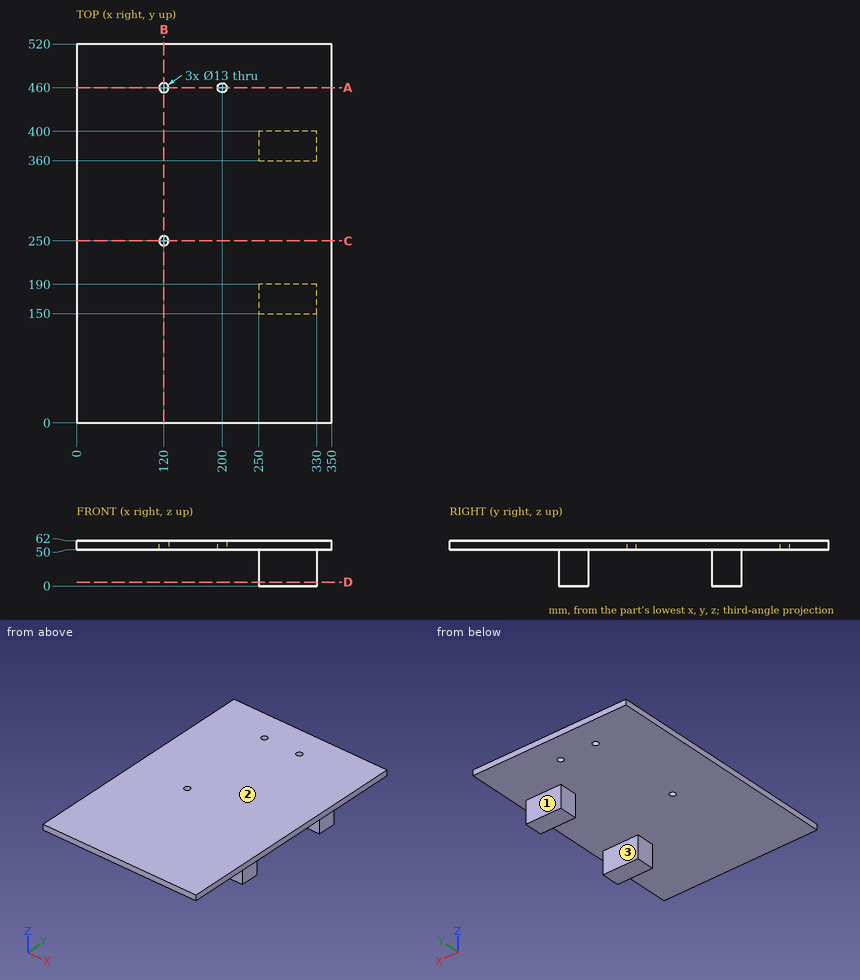
Input: dimensioned drawing with shaded views. Units: mm. Origin: part minimum x, y, z. Round coordinates to 2 decimals unless told otherwise and drop trailing zeros. Loops run counter-clockwise (first coordinate to the right, second up) from the corner with the lowest first, then second, coordinate; pieces in that order, holes last. Notation, with made-up numbers: M -2.75,3 L 50.25,3 A23 ccw 50.25,15 Z; hole C 20.5,-8 d10. An arc over 180 degrees is marked long. Return JSON: item names as keys, results as strings. Group by question number.
1. Section query A-A on y = 460. Output: boundary loops of the cut face in (x, z), and give its area (3 significant figures).
2. Section query B-B on x = 120. Output: boundary loops of the cut face in (y, z), and give its area (3 significant figures).
3. Section query D-D on z = 5.5. Output: boundary loops of the cut face in (x, y), and give its area (3 significant figures).
4. Mould query, pull axis Y, two halves, no side actions, for the marked faces 1, 2 and 3. Classes: released by +Y, released by -Y, zero draft, split by the parting line, or undercut.
5. Section query C-C on y = 250. Output: boundary loops of the cut face in (x, z), and give its area (3 significant figures).
6. Pin query (flat end, axial travel): pin 1 (25 mm diameter, centred on x = 270.5, z = 18, fed in from -Y); pin 2 (12 mm diameter, centred on y = 161.5, z = 14.5, fed in from +X); pin 3 (20 mm diameter, centred on y = 174.5, z = 18.5, fed in from -X); pin 4 (17 mm diameter, centred on x = 120, y = 460, fed in from +Z). Return the tip coordinate at first contact, or that it passes through.
7. Material intervals for line 1 along X through (y, z) = (460, 52); line 2 along Y through (x, z) = (120, 55.25); line 3 along Y through (x, z) = (200, 57), sorted ascending. Write a range as from..to.
Checks:
{
 "1": {"outline": "M 0,50 L 113.5,50 L 113.5,62 L 0,62 Z; M 126.5,50 L 193.5,50 L 193.5,62 L 126.5,62 Z; M 206.5,50 L 350,50 L 350,62 L 206.5,62 Z", "area": "3,890 mm²"},
 "2": {"outline": "M 0,50 L 243.5,50 L 243.5,62 L 0,62 Z; M 256.5,50 L 453.5,50 L 453.5,62 L 256.5,62 Z; M 466.5,50 L 520,50 L 520,62 L 466.5,62 Z", "area": "5,930 mm²"},
 "3": {"outline": "M 250,150 L 330,150 L 330,190 L 250,190 Z; M 250,360 L 330,360 L 330,400 L 250,400 Z", "area": "6,400 mm²"},
 "4": {"face 1": "released by +Y", "face 2": "zero draft", "face 3": "undercut"},
 "5": {"outline": "M 0,50 L 113.5,50 L 113.5,62 L 0,62 Z; M 126.5,50 L 350,50 L 350,62 L 126.5,62 Z", "area": "4,040 mm²"},
 "6": {"pin 1": "stops at y = 150", "pin 2": "stops at x = 330", "pin 3": "stops at x = 250", "pin 4": "stops at z = 62"},
 "7": {"line 1": "x = 0..113.5, 126.5..193.5, 206.5..350", "line 2": "y = 0..243.5, 256.5..453.5, 466.5..520", "line 3": "y = 0..453.5, 466.5..520"}
}
